Source: CAD feature listing. Evaluate the final solid. Frame: model axes, mm. Give positions to 0.01 mm unless a question says otherwise; leave off trailing zeros. Order: outer loops, then holes, each group sorted by start corner. A loop starts at its lowest first (then second) coordinate and runs counter-clockwise, first axis right, second up. Notation, with made-up numbers: (85.25, 37) -> (94.25, 37) arc R17 cw to (94.25, 56) -> close; hole circle Ø8 at (-18.5, 49.5). An arc over 180 degrees is marked (long way). Answer in a Markdown table with one row per item.
```python
from build123d import *

# Parameters (mm, degrees)
SKETCH1_W           = 35
SKETCH1_H           = 12
SKETCH1_R           = 0.8001
SKETCH1_R_2         = 1.4732
BOSS_EXTRUDE1_DEPTH = 0.2


with BuildPart() as part:
    # Sketch1 → Boss-Extrude1 (new body)
    with BuildSketch(Plane.XY):
        with Locations((17.5, -6)):
            Rectangle(SKETCH1_W, SKETCH1_H)
        with Locations((3.5, -8.3)):
            Circle(SKETCH1_R, mode=Mode.SUBTRACT)
        with Locations((5, -4.5)):
            Circle(SKETCH1_R_2, mode=Mode.SUBTRACT)
        with Locations((30, -4.5)):
            Circle(SKETCH1_R_2, mode=Mode.SUBTRACT)
        with Locations((31.5, -8.3)):
            Circle(SKETCH1_R, mode=Mode.SUBTRACT)
        with BuildLine():
            Line((14.522717803, -1.375), (20.477282197, -1.375))
            ThreePointArc((20.477282197, -1.375), (21.05, -1.5), (20.477282197, -1.625))
            Line((20.477282197, -1.625), (14.522717803, -1.625))
            ThreePointArc((14.522717803, -1.625), (13.95, -1.5), (14.522717803, -1.375))
        make_face(mode=Mode.SUBTRACT)
        with BuildLine():
            Line((13.95, -4.5), (13.95, -2.725))
            ThreePointArc((13.95, -2.725), (14.125735931, -2.300735931), (14.55, -2.125))
            Line((14.55, -2.125), (20.45, -2.125))
            ThreePointArc((20.45, -2.125), (20.874264069, -2.300735931), (21.05, -2.725))
            Line((21.05, -2.725), (21.05, -4.5))
            ThreePointArc((21.05, -4.5), (20.520871215, -4.693649167), (20.8, -4.204196011))
            Line((20.8, -4.204196011), (20.8, -2.725))
            ThreePointArc((20.8, -2.725), (20.697487373, -2.477512627), (20.45, -2.375))
            Line((20.45, -2.375), (14.55, -2.375))
            ThreePointArc((14.55, -2.375), (14.302512627, -2.477512627), (14.2, -2.725))
            Line((14.2, -2.725), (14.2, -4.204196011))
            ThreePointArc((14.2, -4.204196011), (14.479128785, -4.693649167), (13.95, -4.5))
        make_face(mode=Mode.SUBTRACT)
    extrude(amount=BOSS_EXTRUDE1_DEPTH)


solid = part.part
```
(1) Section query A-A (x = 5). Return the cut outline in (y, z), plus the area to 3 significant figures.
A:
| item | result |
|---|---|
| outline | (-12, 0) -> (-5.97, 0) -> (-5.97, 0.2) -> (-12, 0.2) -> close; (-3.03, 0) -> (0, 0) -> (0, 0.2) -> (-3.03, 0.2) -> close |
| area | 1.81 mm^2 |
(2) Section query C-C (y = -8). Return the cut outline in (x, z), plus the area to 3 significant figures.
A:
| item | result |
|---|---|
| outline | (0, 0) -> (2.76, 0) -> (2.76, 0.2) -> (0, 0.2) -> close; (4.24, 0) -> (30.76, 0) -> (30.76, 0.2) -> (4.24, 0.2) -> close; (32.24, 0) -> (35, 0) -> (35, 0.2) -> (32.24, 0.2) -> close |
| area | 6.41 mm^2 |
(3) Ray query, probe 1 along Y at (x, z) = (19.5, 0.1) (3 decimals); probe 2 along X at (y, z) = (-3.5, 0.15); probe 3 along Y at (x, z) = (14.25, 0.15). Return the intervals inside material, ascending.
A:
| item | result |
|---|---|
| probe 1 | y = -12 to -2.375, -2.125 to -1.625, -1.375 to 0 |
| probe 2 | x = 0 to 3.92, 6.08 to 13.95, 14.2 to 20.8, 21.05 to 28.92, 31.08 to 35 |
| probe 3 | y = -12 to -4.8, -4.2 to -2.54, -2.21 to -1.8, -1.2 to 0 |
(4) First-contact query: pin 1 Ø2.5 at (x, y) = (30, -4.5) entering from -Z; pin 2 Ø2 at (x, y) = (31.5, -8.3) entering from +Z. Flat tips, straight axial feed; report the tip coordinate or a pass-through.
A:
| item | result |
|---|---|
| pin 1 | passes through |
| pin 2 | stops at z = 0.2 |
(5) Section query B-B (z = 0.05). Return the cut outline in (x, y) (3 decimals), plus the area to 3 significant figures.
A:
| item | result |
|---|---|
| outline | (0, -12) -> (35, -12) -> (35, 0) -> (0, 0) -> close; hole circle Ø1.6 at (3.5, -8.3); hole circle Ø2.946 at (5, -4.5); hole (13.95, -4.5) arc R0.3 ccw (long way) to (14.2, -4.204) -> (14.2, -2.725) arc R0.35 cw to (14.55, -2.375) -> (20.45, -2.375) arc R0.35 cw to (20.8, -2.725) -> (20.8, -4.204) arc R0.3 ccw (long way) to (21.05, -4.5) -> (21.05, -2.725) arc R0.6 ccw to (20.45, -2.125) -> (14.55, -2.125) arc R0.6 ccw to (13.95, -2.725) -> close; hole (14.523, -1.625) -> (20.477, -1.625) arc R0.3 ccw (long way) to (20.477, -1.375) -> (14.523, -1.375) arc R0.3 ccw (long way) to start; hole circle Ø2.946 at (30, -4.5); hole circle Ø1.6 at (31.5, -8.3) |
| area | 397 mm^2 |
